The drawing under review shows one solid part. Ordinate dimensions are in mm from its lowest x, y, z. A direction names the side the tool comes from. Coordinates: 2 decimals unless noted, no trailing zeros. Write each loop counter-clockwise with the first axis right and the second up, starting at its lowest first coordinate (ties: lowest second). Pieces come first, ordered by that corner, then holes. Notation, with made-up numbers: (19, -32) -> (48, -32) arc R23 cw to (48, -20) -> close; hole circle Ø3 at (40, 4). An arc over 180 degrees is marked (long way). Put each result on its own line as item: value. Start each with the question number.
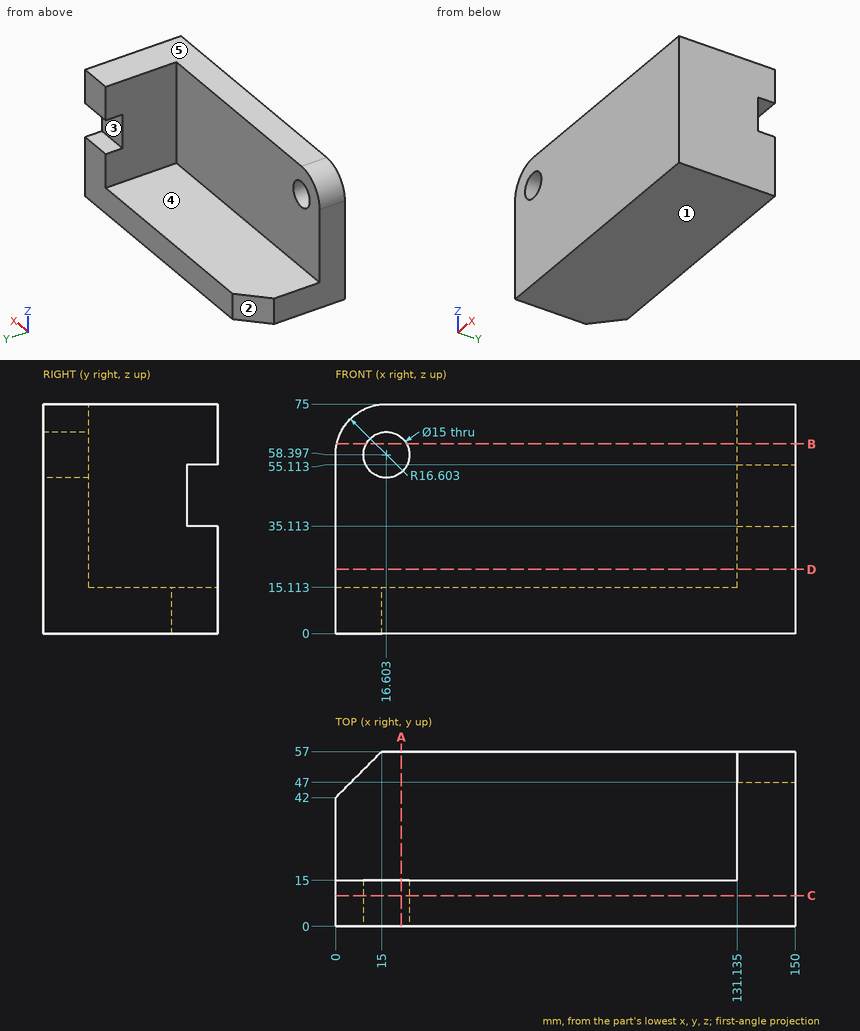
1. Consider section C-C on y = 10. State the section outline as (x, z) points.
2. The part is to be moulded in two halves that separate along Z. For the marked faces 1, 2 and 3, say which applies: released by +Z, released by -Z, zero draft, split by the parting line, or undercut.
3. Wall thickness on line 1 (Z direction, x = 56, y = 51); line 2 (Y direction, x = 80.5, z = 55); line 3 (X direction, y = 50.5, z = 34) (1 decimal): over which ranges is each line inside the solid? List them lowest first. Write a range as from..to.
4. Tool access review of the marked faces 4 and 5: name each direction out of +Z, -Z, +X, -X, +Y, -Y from which nothing blocks a thin tool from reaching the whole face with its end or side.
5. Insertion check: P1, Ø15, axis at x = 141, z = 44.5, coming from the +Y side; P2, Ø2, axis at x = 87, y = 45, coming from the +Z side; P3, Ø3, axis at x = 87.5, z = 38.5, coming from the +Y side; P4, Ø3, axis at y = 50, z = 53.5, coming from the +X side. Each pin has a flat end and moves straight along its axis. Give the tip position at first contact, or say it passes through.
6. Consider section B-B on z = 62. State the section outline as (x, y) points (1 decimal), then the cut area to 3 significant figures.
7. Consider section D-D on z = 21. State the section outline as (x, y) points (1 decimal), then the cut area to 3 significant figures.
8. Consider section A-A on x = 21.5. State the section outline as (y, z) points (1 decimal).
Output values:
1. outline: (0, 0) -> (150, 0) -> (150, 75) -> (16.6, 75) arc R16.6 ccw to (0, 58.4) -> close; hole circle Ø15 at (16.6, 58.4)
2. face 1: released by -Z
2. face 2: zero draft
2. face 3: undercut
3. line 1: z = 0..15.11
3. line 2: y = 0..15
3. line 3: x = 131.1..150
4. face 4: +Z, -X, +Y
4. face 5: +Z, +X, -X, +Y, -Y
5. P1: stops at y = 47
5. P2: stops at z = 15.11
5. P3: stops at y = 15
5. P4: passes through
6. outline: (0.4, 0) -> (10, 0) -> (10, 15) -> (0.4, 15) -> close; (23.2, 0) -> (150, 0) -> (150, 57) -> (131.1, 57) -> (131.1, 15) -> (23.2, 15) -> close
6. area: 2,840 mm^2
7. outline: (0, 0) -> (150, 0) -> (150, 57) -> (131.1, 57) -> (131.1, 15) -> (0, 15) -> close
7. area: 3,040 mm^2
8. outline: (0, 0) -> (57, 0) -> (57, 15.1) -> (15, 15.1) -> (15, 52.7) -> (0, 52.7) -> close; (0, 64.1) -> (15, 64.1) -> (15, 75) -> (0, 75) -> close
